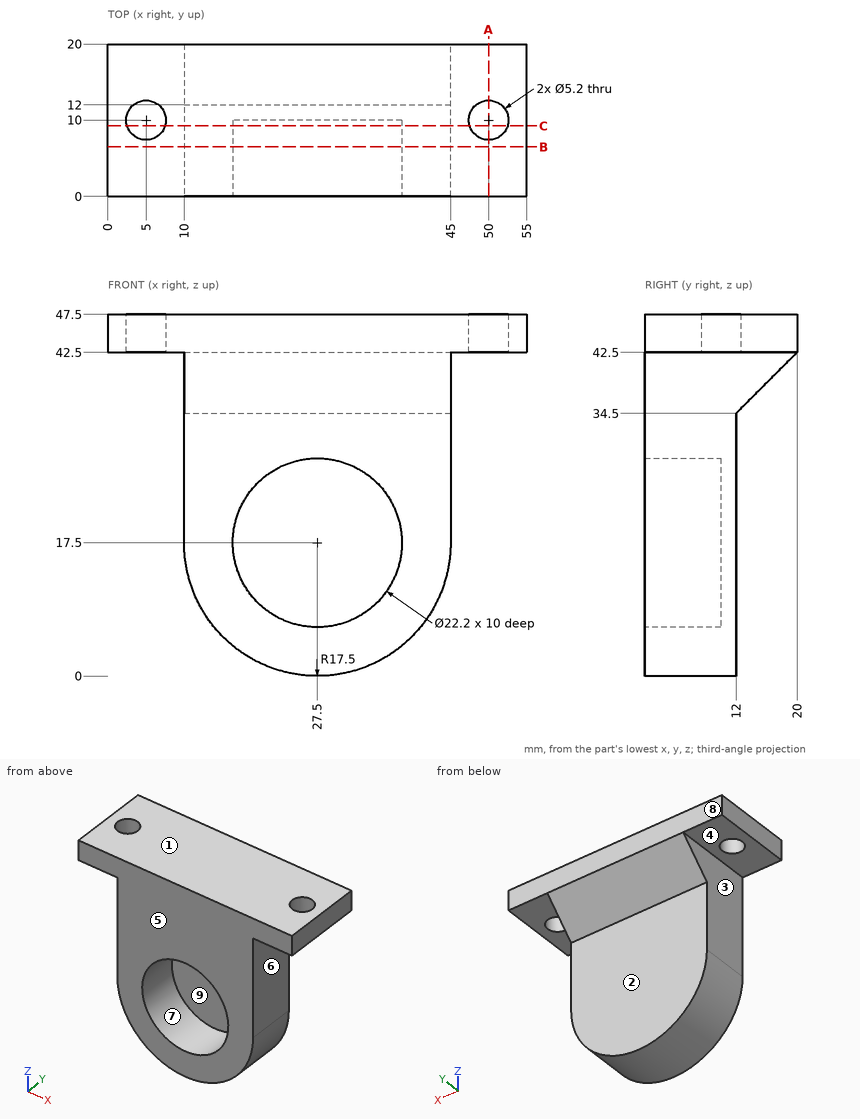
Geometry check sheet. Reference: drawing and pictorial views, mm from the part's lowest x, y, z. A direction names the side the tool comes from. Give positions to 0.01 mm unless a question says otherwise; leave off trailing zeros. Write each loop counter-clockwise with the first axis right and the second up, starting at its lowest first coordinate (ties: lowest second). Pieces come first, ordered by that corner, then holes. Notation, with made-up numbers: (5, -29) -> (40, -29) arc R29 cw to (40, 1) -> close; hole circle Ø1 at (21.25, 83.25). An arc over 180 degrees is marked (long way). One line per item, written item: value. Start each with the question number.
Item 1: Gauge pin test, flat ends, axial feed: pin 1 (17.5 mm diameter, centred on x = 30, z = 11.5, fed in from +Y); pin 2 (5 mm diameter, centred on y = 15, z = 27, fed in from +X); pin 3 (10 mm diameter, centred on y = 6, z = 29.5, fed in from -X); pin 4 (6 mm diameter, centred on x = 5, y = 10, fed in from -Z). Record the tip position at first contact, or that the pin passes through.
Item 2: Section check C-C on y = 9.25. Record the cut outline in (x, z), then the cut area to 3 significant figures.
Item 3: Material ranges on probe 1 along X at (y, z) = (4, 17.5); probe 2 along Y at (x, z) = (5, 43.6); probe 3 along X at (y, z) = (6.25, 31.5), recorded low to high. Write a range as from..to.
Item 4: Section check A-A on x = 50. Record the cut outline in (y, z).
Item 5: Tool access check on the marked faces 1, 2, 3, 4 and 5. Record the directions out of +Z, -Z, +X, -X, +Y, -Y that give a thin tool (end or side, any length) a straight path to the whole face; none if there is none.
Item 6: Section check B-B on y = 6.5. Record the cut outline in (x, z).
Item 7: Draft check along X on the marked faces 6, 7, 8 and 9. Enter one of: +X half, -X half, draft (parallel to the pull), parting line (faces both ways), or undercut.
Results list:
1. pin 1: y = 12
1. pin 2: through
1. pin 3: x = 10
1. pin 4: z = 42.5
2. outline: (0, 42.5) -> (2.51, 42.5) -> (2.51, 47.5) -> (0, 47.5) -> close; (7.49, 42.5) -> (10, 42.5) -> (10, 17.5) arc R17.5 ccw to (45, 17.5) -> (45, 42.5) -> (47.51, 42.5) -> (47.51, 47.5) -> (7.49, 47.5) -> close; (52.49, 42.5) -> (55, 42.5) -> (55, 47.5) -> (52.49, 47.5) -> close; hole circle Ø22.2 at (27.5, 17.5)
2. area: 1,190 mm²
3. probe 1: 10..16.4, 38.6..45
3. probe 2: 0..7.4, 12.6..20
3. probe 3: 10..45
4. outline: (0, 42.5) -> (7.4, 42.5) -> (7.4, 47.5) -> (0, 47.5) -> close; (12.6, 42.5) -> (20, 42.5) -> (20, 47.5) -> (12.6, 47.5) -> close
5. face 1: +Z, +X, -X, +Y, -Y
5. face 2: -Z, +X, -X, +Y
5. face 3: -Z, -X, +Y, -Y
5. face 4: -Z, -X, +Y, -Y
5. face 5: +Z, -Z, +X, -X, -Y
6. outline: (0, 42.5) -> (10, 42.5) -> (10, 17.5) arc R17.5 ccw to (45, 17.5) -> (45, 42.5) -> (55, 42.5) -> (55, 47.5) -> (0, 47.5) -> close; hole circle Ø22.2 at (27.5, 17.5)
7. face 6: +X half
7. face 7: undercut
7. face 8: draft
7. face 9: undercut
